```python
from build123d import *

# Parameters (mm, degrees)
SKETCH1_R           = 6
SKETCH1_R_2         = 5
SKETCH1_R_3         = 3
SKETCH1_R_4         = 4
BOSS_EXTRUDE1_DEPTH = 8


with BuildPart() as part:
    # Sketch1 → Boss-Extrude1 (new body)
    # profile 1 of 3: a face of its own
    with BuildSketch(Plane.XY):
        with BuildLine():
            Line((4, -6.92820323), (4, -85))
            Line((4, -85), (13, -85))
            Line((13, -85), (13, -105))
            Line((13, -105), (-13, -105))
            Line((-13, -105), (-13, -85))
            Line((-13, -85), (-4, -85))
            Line((-4, -85), (-4, -6.92820323))
            ThreePointArc((-4, -6.92820323), (0, 8), (4, -6.92820323))
        make_face()
        with Locations((0, -95)):
            Circle(SKETCH1_R, mode=Mode.SUBTRACT)
        Circle(SKETCH1_R_2, mode=Mode.SUBTRACT)
        with BuildLine():
            Line((-2, -12.430963228), (-2, -81.520541763))
            ThreePointArc((-2, -81.520541763), (-1.707106781, -82.227648544), (-1, -82.520541763))
            Line((-1, -82.520541763), (1, -82.520541763))
            ThreePointArc((1, -82.520541763), (1.707106781, -82.227648544), (2, -81.520541763))
            Line((2, -81.520541763), (2, -12.430963228))
            ThreePointArc((2, -12.430963228), (1.707106781, -11.723856446), (1, -11.430963228))
            Line((1, -11.430963228), (-1, -11.430963228))
            ThreePointArc((-1, -11.430963228), (-1.707106781, -11.723856446), (-2, -12.430963228))
        make_face(mode=Mode.SUBTRACT)
    # profile 2 of 3: a face of its own
    with BuildSketch(Plane.XY):
        Circle(SKETCH1_R_2)
        Circle(SKETCH1_R_3, mode=Mode.SUBTRACT)
    # profile 3 of 3: a face of its own
    with BuildSketch(Plane.XY):
        with Locations((0, -95)):
            Circle(SKETCH1_R)
        with Locations((0, -95)):
            Circle(SKETCH1_R_4, mode=Mode.SUBTRACT)
    extrude(amount=BOSS_EXTRUDE1_DEPTH)


solid = part.part
```
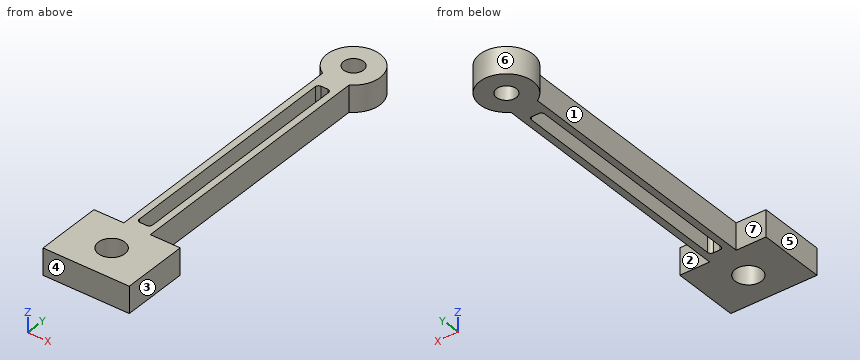
The model under review builds one solid part; all positions refer to its coordinate system, in mm. Face numbers are marked on the shaded views. A direction names the side the tool comes from. Round coordinates to 2 decimals unless told otherwise and drop trailing zeros. Loops run counter-clockwise (first coordinate to the right, second up) from the corner with the lowest first, then second, coordinate; pieces in that order, holes last.
1) Clearance check with flat-ended pins moving along their axes: P1, Ø2.5, axis at x = 10.5, z = 2, coming from the +Y side; P2, Ø4, axis at y = -43, z = 3.5, coming from the -X side; P3, Ø4, axis at x = -8, z = 5, coming from the +Y side. State where each tip first meets the part, or that it passes through.
Values follow:
P1: stops at y = -85
P2: stops at x = -4
P3: stops at y = 5.29
2) Consider section B-B on x = 0. State the section outline as (y, z) points.
Values follow:
outline: (-105, 0) - (-99, 0) - (-99, 8) - (-105, 8) - close; (-91, 0) - (-82.52, 0) - (-82.52, 8) - (-91, 8) - close; (-11.43, 0) - (-3, 0) - (-3, 8) - (-11.43, 8) - close; (3, 0) - (8, 0) - (8, 8) - (3, 8) - close
3) The part is to be moulded in two halves that separate along Y. For the marked faces 4, 5, 6 and 7, say which applies: pulls with the +Y half, pulls with the -Y half, needs draft (parallel to the pull), parting line crosses it, or undercut.
Values follow:
face 4: pulls with the -Y half
face 5: needs draft
face 6: undercut
face 7: undercut
4) Consider section A-A on y = 0. State the section outline as (x, z) points, then the cut area to 3 significant figures.
Values follow:
outline: (-8, 0) - (-3, 0) - (-3, 8) - (-8, 8) - close; (3, 0) - (8, 0) - (8, 8) - (3, 8) - close
area: 80.0 mm2
5) Consider section C-C on z = 2.5. State the section outline as (x, y) points.
Values follow:
outline: (-13, -105) - (13, -105) - (13, -85) - (4, -85) - (4, -6.93) arc R8 ccw (long way) to (-4, -6.93) - (-4, -85) - (-13, -85) - close; hole circle Ø8 at (0, -95); hole circle Ø6 at (0, 0); hole (-2, -81.52) arc R1 ccw to (-1, -82.52) - (1, -82.52) arc R1 ccw to (2, -81.52) - (2, -12.43) arc R1 ccw to (1, -11.43) - (-1, -11.43) arc R1 ccw to (-2, -12.43) - close
6) Tool access review of the marked faces 1, 2 and 3: name each direction out of +Z, -Z, +X, -X, +Y, -Y from which nothing blocks a thin tool from reaching the whole face with its end or side.
Values follow:
face 1: +Z, -Z, -X
face 2: +Z, -Z, +X
face 3: +Z, -Z, +X, +Y, -Y
7) Consider section D-D on y = -33. State the section outline as (x, z) points.
Values follow:
outline: (-4, 0) - (-2, 0) - (-2, 8) - (-4, 8) - close; (2, 0) - (4, 0) - (4, 8) - (2, 8) - close
8) Wall thickness on line 1 along Y through (x, z) = (0, 4.5); line 2 along X through (y, z) = (-64, 1.5); line 3 along Y through (x, z) = (1.25, 7.75): over which ranges is each line inside the solid? List them lowest first.
Values follow:
line 1: y = -105 to -99, -91 to -82.52, -11.43 to -3, 3 to 8
line 2: x = -4 to -2, 2 to 4
line 3: y = -105 to -98.8, -91.2 to -82.49, -11.46 to -2.73, 2.73 to 7.9
